For this review, take the finished solid that the model builds, in its own axes (mm). Face numbers are marked on the shaded views. Round coordinates to 2 decimals unless told otherwise and drop trailing zeros. Order: outer loops, then holes, each group sorted by start corner. A loop starts at its lowest first (then second) coordinate and runs counter-clockwise, first axis right, second up. Notation, with made-up numbers: M 41,43 L 70,43 A32 ccw 70,73 Z; hole C -28,40.5 d1. An arc over 180 degrees is marked long. Put each result on its own line as item: value.
from build123d import *

# Parameters (mm, degrees)
SKETCH1_W           = 41.275
SKETCH1_H           = 41.275
BOSS_EXTRUDE1_DEPTH = 203.2
SKETCH3_R           = 15.875
CUT_EXTRUDE2_DEPTH  = 31.75
SKETCH4_R           = 15.875
CUT_EXTRUDE3_DEPTH  = 209.37411555


with BuildPart() as part:
    # Sketch1 → Boss-Extrude1 (new body)
    with BuildSketch(Plane.XY):
        Rectangle(SKETCH1_W, SKETCH1_H)
    extrude(amount=BOSS_EXTRUDE1_DEPTH)

    # Sketch3 → Cut-Extrude2 (cut)
    with BuildSketch(Plane.XZ.offset(20.6375)):
        with Locations(Location((0, 20.6375, 0), (0, 0, 270))):
            Circle(SKETCH3_R)
    extrude(amount=-CUT_EXTRUDE2_DEPTH, mode=Mode.SUBTRACT)

    # Sketch4 → Cut-Extrude3 (cut, through all)
    with BuildSketch(Plane.ZY.offset(20.6375)):
        with Locations((182.5625, 0)):
            Circle(SKETCH4_R)
    extrude(amount=-CUT_EXTRUDE3_DEPTH, mode=Mode.SUBTRACT)


solid = part.part
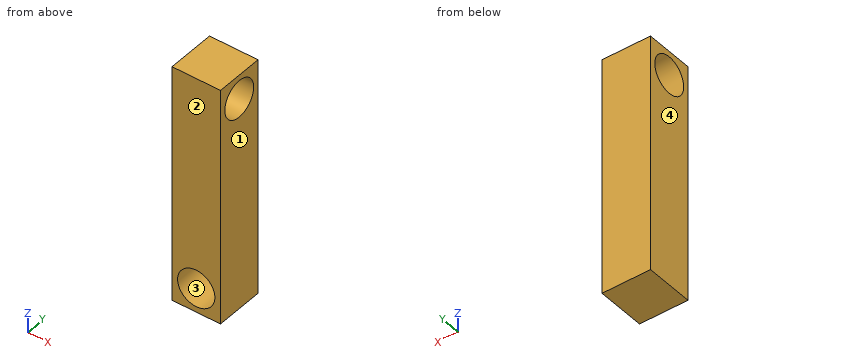
(1) Add section C-C on z = 32.5. Give the boundary of the cut face in (x, y), then the cut area to 3 significant figures.
A:
outline: M -20.64,-20.64 L -10.55,-20.64 L -10.55,11.11 L 10.55,11.11 L 10.55,-20.64 L 20.64,-20.64 L 20.64,20.64 L -20.64,20.64 Z
area: 1,030 mm2
(2) Draft analysis for pull direction X (two halves, no side actions). For the marked faces 1, 2, 3 and 4, state which applies: released by +X, released by -X, zero draft, split by the parting line, or undercut.
A:
face 1: released by +X
face 2: zero draft
face 3: undercut
face 4: released by -X
(3) To check wall thickness, follow L1, parallel to Y at x = 13, z = 183.5; L2, parallel to Z at x = -5, y = 0.5; L3, parallel to Z at x = -3.5, y = 7.5. State the ranges of each line that lie inside material, in increasing order.
A:
L1: y = -20.64 to -15.85, 15.85 to 20.64
L2: z = 0 to 5.57, 35.7 to 166.7, 198.43 to 203.2
L3: z = 0 to 5.15, 36.12 to 168.57, 196.55 to 203.2
(4) Add section A-A on y = 0. State how many separate pieces and enclosed holes the cut face has, then the cut area to 3 significant figures.
A:
separate pieces: 2
enclosed holes: 1
area: 6,280 mm2
